Check sheet for the drawn part. Datum: minimum x, y, z corner. Units: mm. A direction names the side the tool comes from. Round coordinates to 2 decimals unless told otherwise and drop trailing zeros. Write each loop counter-clockwise with the first axis right and the second up, starting at its lowest first coordinate (ties: lowest second). Pieces come first, ordered by that corner, then holes. Notation, with made-up numbers: (87, -29) -> (93, -29) arc R31 cw to (93, -4) -> close; hole circle Ø6 at (56, 82.25). An arc over 180 degrees is marked (long way). Use CSV: the item, a comma, the result in double quotes.
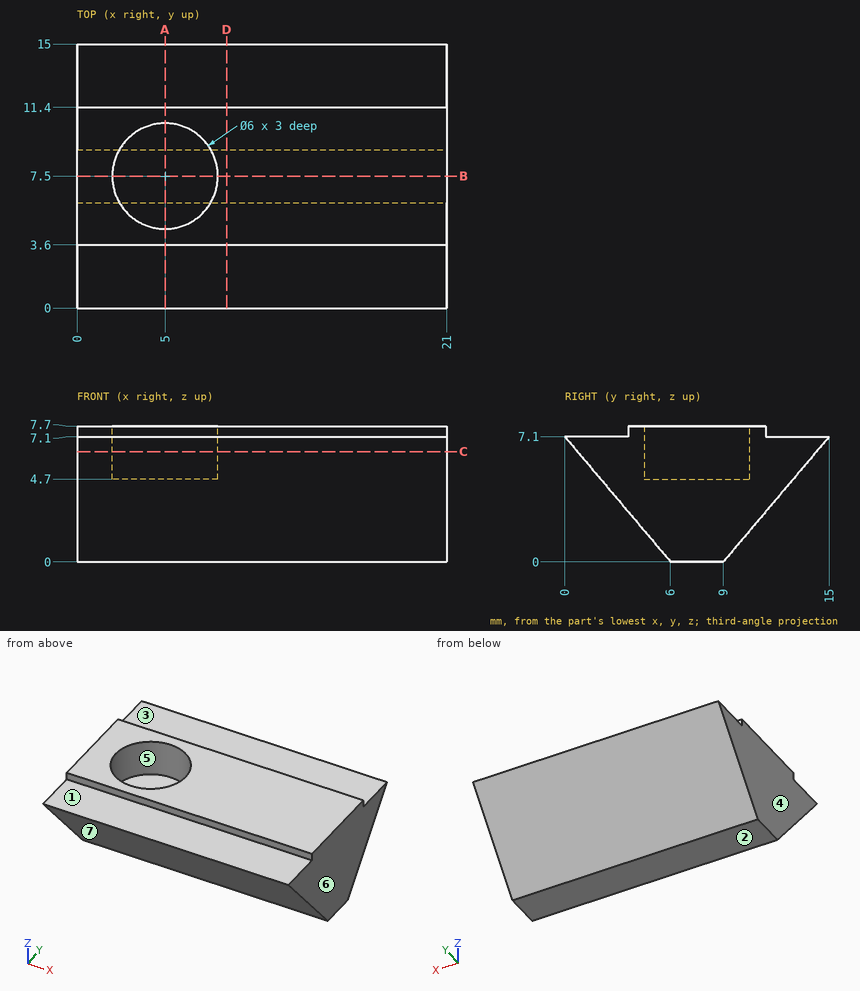
Q1. Section check B-B (y = 7.5). Record the cut outline in (x, z), plus the area to 3 significant figures.
Filled in:
outline,"(0, 0) -> (21, 0) -> (21, 7.7) -> (8, 7.7) -> (8, 4.7) -> (2, 4.7) -> (2, 7.7) -> (0, 7.7) -> close"
area,"144 mm²"
Q2. Go/stop test with flat-tipped pins: P1, Ø4, axis at x = 11.5, y = 13.5, coming from the +Z side; P2, Ø0.7, axis at x = 9.5, z = 7.5, coming from the -Y side. Record where each tip stops, or that it passes through.
Filled in:
P1,"z = 7.1"
P2,"y = 3.6"
Q3. Section check D-D (x = 8.5). Record the cut outline in (y, z), plus the area to 3 significant figures.
Filled in:
outline,"(0, 7.1) -> (6, 0) -> (9, 0) -> (15, 7.1) -> (11.4, 7.1) -> (11.4, 7.7) -> (3.6, 7.7) -> (3.6, 7.1) -> close"
area,"68.6 mm²"
Q4. Material ranges on L1, parallel to X at y = 7.5, z = 5.8; L2, parallel to Y at x = 7.75, z = 5; L3, parallel to X at y = 8.5, z = 6.75, recorded low to high.
Filled in:
L1,"0 to 2, 8 to 21"
L2,"1.77 to 6.3, 8.7 to 13.23"
L3,"0 to 2.17, 7.83 to 21"
Q5. Mould release check, pull along X, two halves, no side actions. Record for the marked faces 4, 5, 6 and 7: released by +X, released by -X, zero draft, split by the parting line, or undercut.
Filled in:
face 4,"released by -X"
face 5,"undercut"
face 6,"released by +X"
face 7,"zero draft"
Q6. Access from +Z, -Z, +X, -X, +Y, -Y to the whole of each face (thin tool, end or side, straight path). Record for the marked faces 1, 2 and 3.
Filled in:
face 1,"+Z, +X, -X, -Y"
face 2,"-Z, +X, -X, +Y, -Y"
face 3,"+Z, +X, -X, +Y"
Q7. Section check C-C (z = 6.25). Record the cut outline in (x, y).
Filled in:
outline,"(0, 0.72) -> (21, 0.72) -> (21, 14.28) -> (0, 14.28) -> close; hole circle Ø6 at (5, 7.5)"
Q8. Section check A-A (x = 5). Record the cut outline in (y, z), plus the area to 3 significant figures.
Filled in:
outline,"(0, 7.1) -> (6, 0) -> (9, 0) -> (15, 7.1) -> (11.4, 7.1) -> (11.4, 7.7) -> (10.5, 7.7) -> (10.5, 4.7) -> (4.5, 4.7) -> (4.5, 7.7) -> (3.6, 7.7) -> (3.6, 7.1) -> close"
area,"50.6 mm²"
